Autodesk Inventor part; units mm, degrees
ref_plane "YZ Plane" through (0, 0, 0) normal (1, 0, 0) x (0, 1, 0)
ref_plane "XZ Plane" through (0, 0, 0) normal (0, 1, 0) x (-1, 0, 0)
ref_plane "XY Plane" through (0, 0, 0) normal (0, 0, 1) x (1, 0, 0)
sketch "Sketch1" plane through (0, 0, 0) normal (0, 1, 0) x (-1, 0, 0)
  circle A0 centre (0, 0) radius 22
  circle A1 centre (0, -22) radius 1.55
  circle A2 centre (0, -22) radius 3
  circle A3 centre (22, 0) radius 3
  circle A4 centre (22, 0) radius 1.55
  circle A5 centre (0, 22) radius 3
  circle A6 centre (0, 22) radius 1.55
  circle A7 centre (-22, 0) radius 3
  circle A8 centre (-22, 0) radius 1.55
  circle A9 centre (0, 0) radius 30
  circle A10 centre (-90, 0) radius 4
  circle A11 centre (-90, 0) radius 15
  line L0 (0, -30) -> (-90, -15)
  line L1 (0, 30) -> (-90, 15)
  circle A12 centre (0, 0) radius 5
  circle A13 centre (0, 0) radius 11
  dimension "d2" = 44
  dimension "d3" = 3.1
  dimension "d4" = 6
  dimension "d5" = 360
  dimension "d6" = 60
  dimension "d8" = 8
  dimension "d9" = 30
  dimension "d10" = 10
  dimension "d11" = 22
extrude "Extrusion1" add sketch "Sketch1" along normal blind 10 contours A0 A4 | A0 A4 | A4 A0 A3 | A0 A3 A4 | A3 A0 A2 A7 A5 | A5 A0 A6 | A0 A6 A5 | A2 A0 A1 | A0 A1 A2 | A6 A0 | A0 A6 | A1 A0 | A0 A1 | A7 A0 A8 | A0 A8 A7 | A8 A0 | A0 A8 | A9 L0 L1 | A9 L0 A11 L1 | A11
sketch "Sketch2" plane through (0, 10, 0) normal (0, 1, 0) x (1, 0, 0)
  circle A0 centre (0, 0) radius 11
  dimension "d14" = 22
extrude "Extrusion2" add sketch "Sketch2" against normal blind 4
Input: part model. Units: mm. Frame: model coordinates. A direction names the side the tool comes from. Round coordinates to 2 decimals unless told otherwise and drop trailing zeros. Loops run counter-clockwise (first coordinate to the right, second up) from the corner with the lowest first, then second, coordinate; pieces in that order, holes last. Notation, with made-up numbers: (9.5, 82.5) -> (21.5, 82.5) arc R12 cw to (21.5, 104.5) -> close; hole circle Ø3 at (-20.75, 19.5). An arc over 180 degrees is marked (long way). Write each question's results on one line, items separated by ' | '.
1. Section A-A (z = 0). Return loops of the section in (x, y), and give its area (3 significant figures).
Geometry results:
outline: (-30, 0) -> (-11, 0) -> (-11, 6) -> (11, 6) -> (11, 0) -> (86, 0) -> (86, 10) -> (-30, 10) -> close; (94, 0) -> (105, 0) -> (105, 10) -> (94, 10) -> close | area: 1,140 mm2
2. Set-up query: faces 1 (the face through (105, 5, 0)), 2 (the face through (2.38, 2.96, 10.74)). Return all of +Z, -Z, +X, -X, +Y, -Y with unobstructed straight access to the full face (end or side cutting, diameter ignored); none if empty.
Geometry results:
face 1: +X, +Y, -Y | face 2: -Y
3. Section C-C (z = 13). Return loops of the section in (x, y).
Geometry results:
outline: (-27.04, 0) -> (97.48, 0) -> (97.48, 10) -> (-27.04, 10) -> close
4. Ray query, line 1 (Z direction, x = 0, y = 4.6); line 2 (Z direction, x = 90, y = 5.75); line 3 (X direction, y = 5.5, z = -1.5). Return the intervals inside material, ascending. Write a range as from..to.
Geometry results:
line 1: -30..-11, 11..30 | line 2: -15..-4, 4..15 | line 3: -29.96..-10.9, 10.9..86.29, 93.71..104.92
5. First-contact query: P1, Ø6.5, axis at x = -4, z = -0.5, coming from the -Y side; P2, Ø5, axis at y = 3.5, z = 6.5, coming from the -X side; P3, Ø3, axis at x = 61, y = 2.5, coming from the +Z side. Flat tips, straight axial feed; report the tip coordinate or a pass-through.
Geometry results:
P1: y = 6 | P2: x = -29.73 | P3: z = 20.08
6. Section B-B (x = 69). Return loops of the section in (y, z), and give its area (3 significant figures).
Geometry results:
outline: (0, -18.5) -> (10, -18.5) -> (10, 18.5) -> (0, 18.5) -> close | area: 370 mm2
